```python
from build123d import *

# Parameters (mm, degrees)
F0_W     = 38.1
F0_H     = 38.1
F1_DEPTH = 38.1
F5_DEPTH = 38.1
F7_DEPTH = 38.1
F8_W     = 25.4
F8_H     = 7.62
F9_DEPTH = 38.1


with BuildPart() as f1:
    # F0 (on Front) → F1 (new body)
    with BuildSketch(Plane.XZ):
        with Locations((19.05, 19.05)):
            Rectangle(F0_W, F0_H)
    extrude(amount=F1_DEPTH)

    # F4 (on face) → F5 (cut)
    with BuildSketch(Plane(origin=(0, 0, 0), x_dir=(-1, 0, 0), z_dir=(0, 1, 0))):
        Polygon((-6.35, 38.1), (-31.75, 38.1), (-26.67, 15.875), (-21.59, 28.575), (-16.51, 28.575), (-11.43, 15.875), align=None)
        Polygon((-31.75, 0), (-38.1, 38.1), (-38.1, 0), align=None)
        Polygon((-19.05, 15.875), (-25.4, 0), (-12.7, 0), align=None)
        Polygon((0, 0), (0, 38.1), (-6.35, 0), align=None)
    extrude(amount=-F5_DEPTH, mode=Mode.SUBTRACT)

    # F6 (on offset) → F7 (cut)
    with BuildSketch(Plane.YZ.offset(38.1)):
        Polygon((-38.1, 38.1), (-38.1, 0), (-31.75, 38.1), align=None)
        Polygon((-19.05, 22.225), (-12.7, 38.1), (-25.4, 38.1), align=None)
        Polygon((-6.35, 38.1), (0, 0), (0, 38.1), align=None)
        Polygon((-31.75, 0), (-6.35, 0), (-11.43, 18.794186), (-16.51, 9.525), (-21.59, 9.525), (-26.67, 18.794186), align=None)
    extrude(amount=-F7_DEPTH, mode=Mode.SUBTRACT)

    # F8 (on offset) → F9 (cut)
    with BuildSketch(Plane.XY.offset(38.1)):
        with Locations((25.4, -11.43)):
            Rectangle(F8_W, F8_H)
        with Locations((12.7, -26.67)):
            Rectangle(F8_W, F8_H)
    extrude(amount=-F9_DEPTH, mode=Mode.SUBTRACT)


solid = f1.part
```
The model under review builds one solid part; all positions refer to its coordinate system, in mm. A direction names the side the tool comes from. Coordinates: 2 decimals unless noted, no trailing zeros. Write each loop counter-clockwise with the first axis right and the second up, starting at its lowest first coordinate (ties: lowest second). Pieces come first, ordered by that corner, then holes.
1) We need section A-A on y = -26. State the section outline as (x, z) points, then the cut area to 3 significant figures.
2) Clearance check with flat-ended pins moving along their axes: pin 1 Ø8.5 at (y, z) = (-28, 13.5) entering from -X; pin 2 Ø0.6 at (x, y) = (19.5, -22) entering from +Z (3 decimals); pin 3 Ø8 at (x, z) = (11, 9.5) entering from -Y. State where each tip first meets the part, or that it passes through.
3) The part is to be moulded in two halves that separate along Y. For faces 5 (the face through (19.32, -3.22, 19.32)), 6 (the face through (29.45, -24.09, 14.09)), 7 (the face through (15.83, -4.6, 7.83)), say which applies: pulls with the +Y half, pulls with the -Y half, needs draft (parallel to the pull), parting line crosses it, or undercut.
4) To check wall thickness, follow probe 1 along Y at (x, z) = (5.5, 13); probe 2 along X at (y, z) = (-31, 17.5); probe 3 along X at (y, z) = (-17.5, 17). State the ranges of each line that lie inside material, in increasing order.
5) Machinability: for faces 1 (the face through (20.302, -18.997, 12.744)), 2 (the face through (33.18, -22.27, 30.27)), 3 (the face through (10.998, -22.216, 10.667)), 4 (the face through (25.4, -28, 15)), which of the approach directions +Z, -Z, +X, -X, +Y, -Y give a long, thin tool a straight path to every point of the face, cutting with its end or side? Answer none if there is none.
6) We need section D-D on z = 3. State the section outline as (x, y) points, then the cut area to 3 significant figures.
7) We need section B-B on z = 11. State the section outline as (x, y) points.
Answer list:
1. outline: (25.4, 17.57) - (25.99, 17.57) - (25.4, 19.05) - close; (27.06, 17.57) - (34.68, 17.57) - (38.1, 38.1) - (31.75, 38.1) - close
1. area: 144 mm2
2. pin 1: stops at x = 3.52
2. pin 2: stops at z = 28.575
2. pin 3: stops at y = -37.18
3. face 5: pulls with the +Y half
3. face 6: undercut
3. face 7: needs draft
4. probe 1: y = -35.93 to -30.48, -22.86 to -14.61, -9.86 to -2.17
4. probe 2: x = 3.43 to 11.06, 12.08 to 26.02, 27.04 to 34.67
4. probe 3: x = 3.52 to 11.17, 11.88 to 26.22, 26.93 to 34.58
5. face 1: -Z, +Y, -Y
5. face 2: +Z, +X, -X
5. face 3: -Z, +X, -X
5. face 4: +Z, -Z, -X
6. outline: (5.85, -37.6) - (13.9, -37.6) - (13.9, -30.94) - (5.85, -30.94) - close; (5.85, -7.16) - (13.9, -7.16) - (13.9, -0.5) - (5.85, -0.5) - close; (24.2, -37.6) - (32.25, -37.6) - (32.25, -30.94) - (24.2, -30.94) - close; (24.2, -7.16) - (32.25, -7.16) - (32.25, -0.5) - (24.2, -0.5) - close
6. area: 214 mm2
7. outline: (4.52, -36.27) - (17.1, -36.27) - (17.1, -30.48) - (4.52, -30.48) - close; (4.52, -22.4) - (17.1, -22.4) - (17.1, -15.7) - (4.52, -15.7) - close; (4.52, -9.32) - (12.7, -9.32) - (12.7, -7.62) - (17.1, -7.62) - (17.1, -1.83) - (4.52, -1.83) - close; (21, -36.27) - (33.58, -36.27) - (33.58, -28.78) - (25.4, -28.78) - (25.4, -30.48) - (21, -30.48) - close; (21, -22.4) - (33.58, -22.4) - (33.58, -15.7) - (21, -15.7) - close; (21, -7.62) - (33.58, -7.62) - (33.58, -1.83) - (21, -1.83) - close
